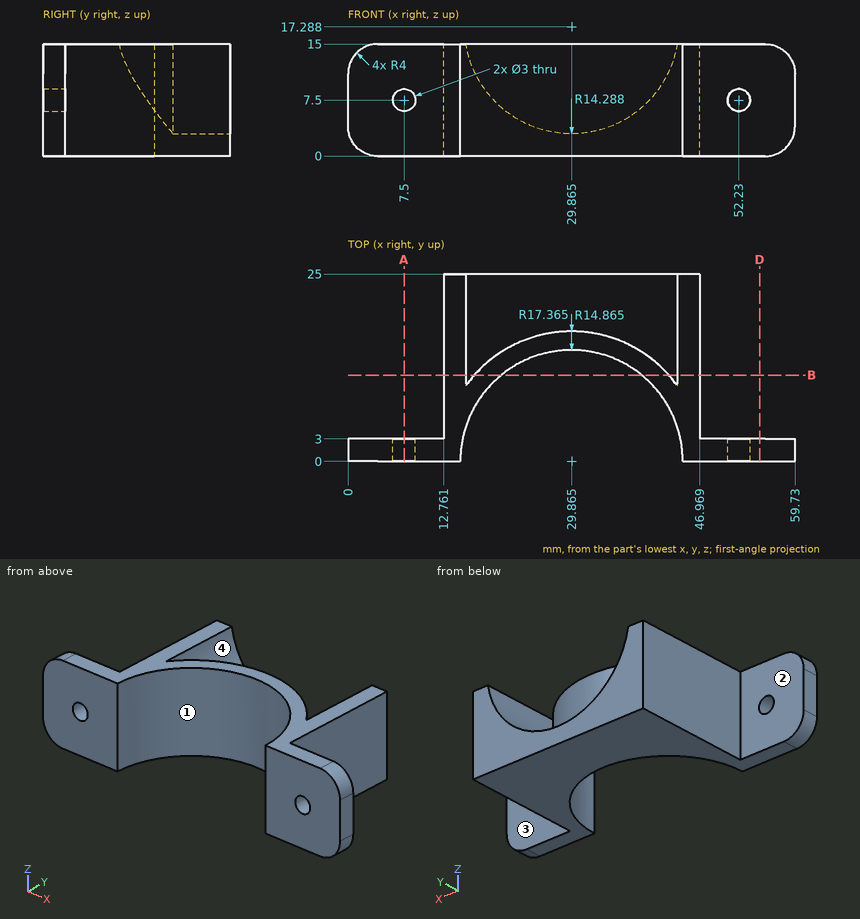
Answer from the drawing. Dimensions are ordinates in mm from the lowest x, y and z of the part. A direction names the side the tool comes from. Round coordinates to 2 decimals unless told otherwise and drop trailing zeros. Write each loop counter-clockwise with the first axis right and the second up, starting at its lowest first coordinate (ties: lowest second). Pieces come first, ordered by that corner, then holes. Notation, with made-up numbers: M 86.25,77 L 128.25,77 A24 cw 128.25,108 Z; hole C -13,13 d9. An arc over 180 degrees is marked long. Write each question's results on one line, items separated by ' | '. Start each with the question number.
Item 1: Given pin 1 Ø8 at (x, z) = (38, 8.5) entering from -Y (1 decimal); pin 2 Ø8 at (x, z) = (51, 11) entering from +Y; pin 3 Ø7.5 at (y, z) = (10, 4) entering from -X, each flat-ended and moving along its own axis, determine where each tip first touches the part or whether it passes through.
Item 2: Find section D-D on x = 55. Write down the section's boundary in (y, z), and give its area (3 significant figures).
Item 3: Find section B-B on y = 11.5. Write down the section's boundary in (x, z) (1 decimal), and give its area (3 significant figures).
Item 4: Find section A-A on x = 7.5. Write down the section's boundary in (y, z), and give its area (3 significant figures).
Item 5: Straight lines are drawn through the part: probe 1 along Z at (x, y) = (52.23, 0.8); probe 2 along X at (y, z) = (2.2, 7.5); probe 3 along X at (y, z) = (1.75, 7.5). For each, find the intervals that lie inside material, in ascending order.
Item 6: Which of the six approach directions +Z, -Z, +X, -X, +Y, -Y give full straight-line access (tool end or side, diameter ignored) to the marked faces 1, 2, 3 and 4?
Answer block:
1) pin 1: stops at y = 8.6 | pin 2: stops at y = 3 | pin 3: stops at x = 12.76
2) outline: M 0,0 L 3,0 L 3,15 L 0,15 Z | area: 45.0 mm²
3) outline: M 12.8,0 L 20.4,0 L 20.4,15 L 16.9,15 L 16.9,11.4 A14.3 cw 15.8,15 L 12.8,15 Z; M 39.3,0 L 47,0 L 47,15 L 44,15 A14.3 cw 42.9,11.4 L 42.9,15 L 39.3,15 Z | area: 226 mm²
4) outline: M 0,0 L 3,0 L 3,6 L 0,6 Z; M 0,9 L 3,9 L 3,15 L 0,15 Z | area: 36.0 mm²
5) probe 1: z = 0 to 6, 9 to 15 | probe 2: x = 0 to 6, 9 to 15.16, 44.57 to 50.73, 53.73 to 59.73 | probe 3: x = 0 to 6, 9 to 15.1, 44.63 to 50.73, 53.73 to 59.73
6) face 1: +Z, -Z, -Y | face 2: +Z, -Z, -X, +Y | face 3: +Z, -Z, +X, +Y | face 4: +Z, +Y
